Part model, mm, in its own coordinate system. Face numbers are marked on the shaded views. A direction names the side the tool comes from. Round coordinates to 2 decimals unless told otherwise and drop trailing zeros. Order: outer loops, then holes, each group sorted by start corner. A loop starts at its lowest first (then second) coordinate and runs counter-clockwise, first axis right, second up. Notation, with made-up numbers: M 62,-15 L 87,-15 A20 ccw 87,15 Z; hole C 13,-37 d5. An arc over 180 degrees is marked long. One line per question, with ' | ' between items.
from build123d import *

# Parameters (mm, degrees)
SHAFT_MOUNT_SKETCH_R           = 52.5
SHAFT_MOUNT_SKETCH_R_2         = 40.5
CYLINDRICAL_BORE_EXTRUDE_DEPTH = 63
SKETCH1_3_R                    = 23.665
SKETCH1_3_R_2                  = 11.665
BOLT_HOLES_EXTRUDE_DEPTH       = 25
BOLT_HOLES_EXTRUDE_2_DEPTH     = 25
SHAFT_MOUNT_GUSSETS_DEPTH      = 12
FLANGE_START                   = 12
FLANGE_EXTRUDED_CUT_1_DEPTH    = 3
FLANGE_EXTRUDED_CUT_2_DEPTH    = 3


with BuildPart() as part:
    # Shaft Mount Sketch → Cylindrical Bore Extrude (new body)
    with BuildSketch(Plane.XY):
        Circle(SHAFT_MOUNT_SKETCH_R)
        Circle(SHAFT_MOUNT_SKETCH_R_2, mode=Mode.SUBTRACT)
    extrude(amount=CYLINDRICAL_BORE_EXTRUDE_DEPTH)



with BuildPart() as body_2:
    # Sketch1<3> → Bolt Holes Extrude (new body)
    with BuildSketch(Plane.XY):
        with Locations((-87.5, 0)):
            Circle(SKETCH1_3_R)
        with Locations((-87.5, 0)):
            Circle(SKETCH1_3_R_2, mode=Mode.SUBTRACT)
    extrude(amount=BOLT_HOLES_EXTRUDE_DEPTH)


with BuildPart() as body_3:
    # Sketch1<3> → Bolt Holes Extrude 2 (new body)
    with BuildSketch(Plane.XY):
        with Locations((87.5, 0)):
            Circle(SKETCH1_3_R)
        with Locations((87.5, 0)):
            Circle(SKETCH1_3_R_2, mode=Mode.SUBTRACT)
    extrude(amount=BOLT_HOLES_EXTRUDE_2_DEPTH)


with BuildPart() as part_1:
    add(part.part)

    add(body_2.part)  # Shaft Mount Gussets merges body 2

    add(body_3.part)  # Shaft Mount Gussets merges body 3
    # Sketch1<4> → Shaft Mount Gussets (add)
    with BuildSketch(Plane.XY):
        with BuildLine():
            Line((-18.179450038, 49.251980634), (-87.5, 23.665))
            ThreePointArc((-87.5, 23.665), (-63.835, 0), (-87.5, -23.665))
            Line((-87.5, -23.665), (-18.179450038, -49.251980634))
            ThreePointArc((-18.179450038, -49.251980634), (-52.5, 0), (-18.179450038, 49.251980634))
        make_face()
        with BuildLine():
            Line((87.5, 23.665), (18.179450038, 49.251980634))
            ThreePointArc((18.179450038, 49.251980634), (52.5, 0), (18.179450038, -49.251980634))
            Line((18.179450038, -49.251980634), (87.5, -23.665))
            ThreePointArc((87.5, -23.665), (63.835, 0), (87.5, 23.665))
        make_face()
    extrude(amount=SHAFT_MOUNT_GUSSETS_DEPTH)

    # Socket Sketch<6> → Flange Extruded Cut 1 (cut)
    with BuildSketch(Plane.XY.offset(FLANGE_START)):
        with BuildLine():
            ThreePointArc((53.167380744, -33.139708031), (49.854923731, -32.28250119), (49.5, -28.879384358))
            ThreePointArc((49.5, -28.879384358), (56.918852132, 0), (49.5, 28.879384358))
            ThreePointArc((49.5, 28.879384358), (49.854923731, 32.28250119), (53.167380744, 33.139708031))
            Line((53.167380744, 33.139708031), (72.424639318, 26.031641195))
            ThreePointArc((72.424639318, 26.031641195), (74.376149951, 23.457842629), (72.861251786, 20.605139287))
            ThreePointArc((72.861251786, 20.605139287), (60.835, 0), (72.861251786, -20.605139287))
            ThreePointArc((72.861251786, -20.605139287), (74.376149951, -23.457842629), (72.424639318, -26.031641195))
            Line((72.424639318, -26.031641195), (53.167380744, -33.139708031))
        make_face()
    extrude(amount=-FLANGE_EXTRUDED_CUT_1_DEPTH, mode=Mode.SUBTRACT)

    # Socket Sketch<7> → Flange Extruded Cut 2 (cut)
    with BuildSketch(Plane.XY.offset(FLANGE_START)):
        with BuildLine():
            ThreePointArc((-49.5, 28.879384358), (-56.918852132, 0), (-49.5, -28.879384358))
            ThreePointArc((-49.5, -28.879384358), (-49.854923731, -32.28250119), (-53.167380744, -33.139708031))
            Line((-53.167380744, -33.139708031), (-72.424639318, -26.031641195))
            ThreePointArc((-72.424639318, -26.031641195), (-74.376149951, -23.457842629), (-72.861251786, -20.605139287))
            ThreePointArc((-72.861251786, -20.605139287), (-60.835, 0), (-72.861251786, 20.605139287))
            ThreePointArc((-72.861251786, 20.605139287), (-74.376149951, 23.457842629), (-72.424639318, 26.031641195))
            Line((-72.424639318, 26.031641195), (-53.167380744, 33.139708031))
            ThreePointArc((-53.167380744, 33.139708031), (-49.854923731, 32.28250119), (-49.5, 28.879384358))
        make_face()
    extrude(amount=-FLANGE_EXTRUDED_CUT_2_DEPTH, mode=Mode.SUBTRACT)


solid = part_1.part
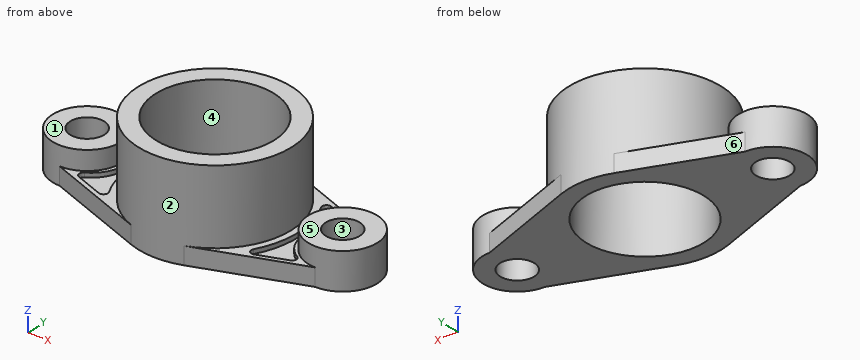
1) Probe line 1 (Y direction, x = 87.5, z = 16.5) (3 decimals); line 2 (Y direction, x = 0, z = 27); line 3 (X direction, y = -17, z = 57). List the from-to ranges inside material, lowest first. Write a range as [from, to].
The answers:
line 1: y = [-23.665, -11.665], [11.665, 23.665] | line 2: y = [-52.5, -40.5], [40.5, 52.5] | line 3: x = [-49.67, -36.76], [36.76, 49.67]
2) Saw through at A-A (x = 0). List the corners of the cut face in (y, z), plus the area to 3 significant figures.
The answers:
outline: M -52.5,0 L -40.5,0 L -40.5,63 L -52.5,63 Z; M 40.5,0 L 52.5,0 L 52.5,63 L 40.5,63 Z | area: 1,510 mm²
3) Drop flat-ended pins along their axis: pin 1 (2 mm diameter, centred on x = 20, z = 20, fed in from -Y); pin 2 (1 mm diameter, centred on y = -30.5, z = 51, fed in from +X); pin 3 (4 mm diameter, centred on x = 19, z = 51, fed in from +Y); pin 4 (3 mm diameter, centred on x = -13, y = 38, fed in from -Z). Give the stop position or say it passes through.
The answers:
pin 1: stops at y = -48.94 | pin 2: stops at x = 43.08 | pin 3: stops at y = 49.67 | pin 4: stops at z = 0
4) Saw through at C-C (y = 0). Give the number of separate pieces and of enclosed holes in the cut face, plus the area to 3 significant figures.
The answers:
separate pieces: 4 | enclosed holes: 0 | area: 2,960 mm²
5) Saw through at D-D (x = -35.5). List the corners of the cut face in (y, z), plus the area to 3 significant figures.
The answers:
outline: M -42.86,0 L -19.49,0 L -19.49,63 L -38.68,63 L -38.68,12 L -42.86,12 Z; M 19.49,0 L 42.86,0 L 42.86,12 L 38.68,12 L 38.68,63 L 19.49,63 Z | area: 2,520 mm²
6) Which spindle directions (+Z, -Z, +X, -X, +Y, -Y) get a long thin tool onto all of the face, cutting with end or side? Do the marked faces 1, 2 and 3. Say none if no direction does.
The answers:
face 1: +Z, -X, +Y, -Y | face 2: +Z | face 3: +Z, -Z
7) Two-plate mould, pull along X, no slides. Class the marked faces 4, 5 and 6: released by +X, released by -X, zero draft, split by the parting line, or undercut.
The answers:
face 4: undercut | face 5: zero draft | face 6: released by -X
8) Saw through at B-B (z = 19.5). List the corners of the cut face in (x, y) (3 decimals).
The answers:
outline: C -87.5,0 d47.33; C 0,0 d105; C 87.5,0 d47.33; hole C -87.5,0 d23.33; hole C 0,0 d81; hole C 87.5,0 d23.33
